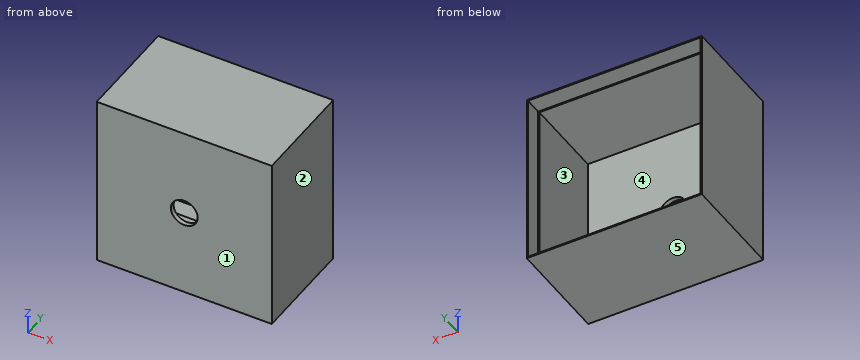
```python
from build123d import *

# Parameters (mm, degrees)
F0_W     = 76.2
F0_H     = 76.2
F1_DEPTH = 38.1
F2_W     = 74.168
F2_H     = 74.168
F3_DEPTH = 36.068
F4_W     = 75.2094
F4_H     = 75.2094
F4_W_2   = 76.2
F4_H_2   = 76.2
F5_DEPTH = 7.62
F6_R     = 5.840403
F7_DEPTH = 12.7


with BuildPart() as f1:
    # F0 (on Front) → F1 (new body)
    with BuildSketch(Plane.XZ):
        Rectangle(F0_W, F0_H)
    extrude(amount=F1_DEPTH)

    # F2 (on face) → F3 (cut)
    with BuildSketch(Plane(origin=(0, 0, 0), x_dir=(-1, 0, 0), z_dir=(0, 1, 0))):
        Rectangle(F2_W, F2_H)
    extrude(amount=-F3_DEPTH, mode=Mode.SUBTRACT)

    # F4 (on face) → F5 (join)
    with BuildSketch(Plane(origin=(0, 0, 0), x_dir=(-1, 0, 0), z_dir=(0, 1, 0))):
        Rectangle(F4_W, F4_H)
        Rectangle(F4_W_2, F4_H_2)
        Rectangle(F4_W, F4_H, mode=Mode.SUBTRACT)
    extrude(amount=F5_DEPTH)

    # F6 (on face) → F7 (cut)
    with BuildSketch(Plane.XZ.offset(38.1)):
        Circle(F6_R)
    extrude(amount=-F7_DEPTH, mode=Mode.SUBTRACT)


solid = f1.part
```
Here's how the part is built. I have some questions about the finished solid (model axes, mm). Face numbers are marked on the shaded views. A direction names the side the tool comes from. Give positions to 0.01 mm unless a question says otherwise; leave off trailing zeros. Loops run counter-clockwise (first coordinate to the right, second up) from the corner with the lowest first, then second, coordinate; pieces in that order, holes last. Notation, with made-up numbers: M 85,-37.75 L 125,-37.75 A23 cw 125,-12.75 Z; hole C 32.5,-4 d1. An arc over 180 degrees is marked long. Return JSON: item names as keys, results as strings.
Item 1: I'm going to push a flat-ended pin straight in: pin 1 Ø2 at (x, z) = (0, -24.5) entering from +Y. Where does the tip first touch, or does it pass through?
A:
{"pin 1": "stops at y = -36.07"}
Item 2: Imagine slicing it at C-C on y = 2.5. List the corners of the cut face in (x, z) for me, then the cut area to 3 significant figures.
A:
{"outline": "M -38.1,-38.1 L 38.1,-38.1 L 38.1,38.1 L -38.1,38.1 Z; hole M -37.6,-37.6 L 37.6,-37.6 L 37.6,37.6 L -37.6,37.6 Z", "area": "150 mm^2"}
Item 3: Please list where these lines run through material, in increasing order: line 1 (X direction, y = 2, z = -3.5); line 2 (Z direction, x = 0, y = -37); line 3 (Z direction, x = -32.5, y = -18.5).
A:
{"line 1": "x = -38.1 to -37.6, 37.6 to 38.1", "line 2": "z = -38.1 to -5.84, 5.84 to 38.1", "line 3": "z = -38.1 to -37.08, 37.08 to 38.1"}
Item 4: On a 3-axis mill with a long thin cutter (end or side, diameter ignored), from which of +Z, -Z, +X, -X, +Y, -Y can I reach the whole of each face in a straight line? I mean the marked faces 4 and 5. Say none if no direction works.
A:
{"face 4": "+Y", "face 5": "-Z, +X, -X, +Y, -Y"}
Item 5: Imagine slicing it at B-B on z = 0. List the corners of the cut face in (x, y) for me, then the cut area to 3 significant figures.
A:
{"outline": "M -38.1,-38.1 L -5.84,-38.1 L -5.84,-36.07 L -37.08,-36.07 L -37.08,0 L -37.6,0 L -37.6,7.62 L -38.1,7.62 Z; M 5.84,-38.1 L 38.1,-38.1 L 38.1,7.62 L 37.6,7.62 L 37.6,0 L 37.08,0 L 37.08,-36.07 L 5.84,-36.07 Z", "area": "212 mm^2"}
Item 6: Imagine slicing it at D-D on z = -15. List the corners of the cut face in (x, y) for me.
A:
{"outline": "M -38.1,-38.1 L 38.1,-38.1 L 38.1,7.62 L 37.6,7.62 L 37.6,0 L 37.08,0 L 37.08,-36.07 L -37.08,-36.07 L -37.08,0 L -37.6,0 L -37.6,7.62 L -38.1,7.62 Z"}
Item 7: Thinking about a two-plate mould opening in X: for the marked faces 1, 2 and 3, which applies, released by +X, released by -X, zero draft, split by the parting line, or undercut?
A:
{"face 1": "zero draft", "face 2": "released by +X", "face 3": "undercut"}
Item 8: Imagine slicing it at A-A on x = 0. List the corners of the cut face in (y, z) for me, then the cut area to 3 significant figures.
A:
{"outline": "M -38.1,-38.1 L 7.62,-38.1 L 7.62,-37.6 L 0,-37.6 L 0,-37.08 L -36.07,-37.08 L -36.07,-5.84 L -38.1,-5.84 Z; M -38.1,5.84 L -36.07,5.84 L -36.07,37.08 L 0,37.08 L 0,37.6 L 7.62,37.6 L 7.62,38.1 L -38.1,38.1 Z", "area": "212 mm^2"}
